Check sheet for the modelled part. Datum: model origin and axes. Units: mm. Round coordinates to 2 decimals unless told otherwise and drop trailing zeros. Order: outer loops, then holes, each group sorted by start corner. A loop starts at its lowest first (then second) coordinate and runs counter-clockwise, first axis right, second up.
```python
from build123d import *

# Parameters (mm, degrees)
SKETCH2_W           = 19.05
SKETCH2_H           = 9.525
BOSS_EXTRUDE1_DEPTH = 3.175
SKETCH3_R           = 0.79375
CUT_EXTRUDE1_DEPTH  = 12.1125
FILLET1_R           = 0.396875


with BuildPart() as part:
    # Sketch2 → Boss-Extrude1 (new body)
    with BuildSketch(Plane.XY):
        Rectangle(SKETCH2_W, SKETCH2_H)
    extrude(amount=BOSS_EXTRUDE1_DEPTH)

    # Sketch3 → Cut-Extrude1 (cut, through all)
    with BuildSketch(Plane.XY.offset(3.175)):
        with Locations((-7.9375, 3.175)):
            Circle(SKETCH3_R)
        with Locations(Location((-7.9375, -3.175, 0), (0, 0, 180))):
            Circle(SKETCH3_R)
        with Locations((7.9375, -3.175)):
            Circle(SKETCH3_R)
        with Locations(Location((7.9375, 3.175, 0), (0, 0, 180))):
            Circle(SKETCH3_R)
    extrude(amount=-CUT_EXTRUDE1_DEPTH, mode=Mode.SUBTRACT)

    # Fillet1
    fillet1_edges = [part.edges().sort_by_distance(p)[0] for p in [
        (9.525, -4.7625, 1.5875),
        (-9.525, -4.7625, 1.5875),
        (-9.525, 4.7625, 1.5875),
        (9.525, 4.7625, 1.5875),
    ]]
    fillet(fillet1_edges, radius=FILLET1_R)


solid = part.part
```
Item 1: Sectioned sample at C-C (z = 2.6). Record the cut outline in (x, y) (1 decimal).
Answer:
outline: (-9.5, -4.4) arc R0.4 ccw to (-9.1, -4.8) - (9.1, -4.8) arc R0.4 ccw to (9.5, -4.4) - (9.5, 4.4) arc R0.4 ccw to (9.1, 4.8) - (-9.1, 4.8) arc R0.4 ccw to (-9.5, 4.4) - close; hole circle Ø1.6 at (-7.9, -3.2); hole circle Ø1.6 at (-7.9, 3.2); hole circle Ø1.6 at (7.9, -3.2); hole circle Ø1.6 at (7.9, 3.2)
Item 2: Release check for a two-part mould opening along Y. For faces 1 (the cylindrical face through (-7.77, -2.4, 1.61)), 2 (the flat face through (0, -4.762, 2)), 3 (the flat face through (0, 0, 3.175)) record: released by +Y, released by -Y, zero draft, split by the parting line, or undercut.
Answer:
face 1: undercut
face 2: released by -Y
face 3: zero draft
Item 3: Go/stop test with a flat-tipped pin: P1, Ø1.4, axis at x = 7.94, y = -3.18, coming from the +Z side. Record where the tip stops, or that it passes through.
Answer:
P1: passes through
Item 4: Sectioned sample at B-B (x = 8.25). Record the cut outline in (y, z) (1 decimal).
Answer:
outline: (-4.8, 0) - (-3.9, 0) - (-3.9, 3.2) - (-4.8, 3.2) - close; (-2.4, 0) - (2.4, 0) - (2.4, 3.2) - (-2.4, 3.2) - close; (3.9, 0) - (4.8, 0) - (4.8, 3.2) - (3.9, 3.2) - close
Item 5: Sectioned sample at A-A (y = 3). Record the cut outline in (x, z) (3 decimals), and give its area (3 significant figures).
Answer:
outline: (-9.525, 0) - (-8.712, 0) - (-8.712, 3.175) - (-9.525, 3.175) - close; (-7.163, 0) - (7.163, 0) - (7.163, 3.175) - (-7.163, 3.175) - close; (8.712, 0) - (9.525, 0) - (9.525, 3.175) - (8.712, 3.175) - close
area: 50.7 mm2
Item 6: Scan lines: line 1 along X through (y, z) = (-3.75, 0.2) (3 decimals); line 2 along Y through (x, z) = (-8.5, 0.7); line 3 along Y through (x, z) = (-8.25, 0.9). Record each from-to range of solid material in increasing order.
Answer:
line 1: x = -9.525 to -8.485, -7.39 to 7.39, 8.485 to 9.525
line 2: y = -4.76 to -3.74, -2.61 to 2.61, 3.74 to 4.76
line 3: y = -4.76 to -3.9, -2.45 to 2.45, 3.9 to 4.76
